Geometry: final body of the model. Coordinates: model frame, mm. Face numbers are marked on the shaded views. A direction names the side the tool comes from. Coordinates: 2 decimals unless noted, no trailing zeros. Write each loop counter-clockwise with the first axis right and the second up, starting at its lowest first coordinate (ties: lowest second). Pieces come first, ordered by that corner, then holes.
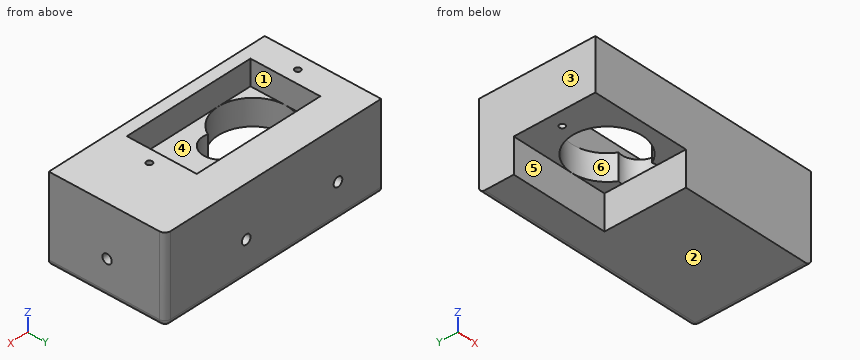
Autodesk Inventor part; units mm, degrees
ref_plane "YZ Plane" through (0, 0, 0) normal (1, 0, 0) x (0, 1, 0)
ref_plane "XZ Plane" through (0, 0, 0) normal (0, 1, 0) x (-1, 0, 0)
ref_plane "XY Plane" through (0, 0, 0) normal (0, 0, 1) x (1, 0, 0)
sketch "Sketch1" plane through (0, 0, 0) normal (0, 0, 1) x (1, 0, 0)
  line L0 (0, 0) -> (-40, 0)
  line L1 (-40, 0) -> (-40, -18)
  line L2 (-40, -18) -> (0, -18)
  line L3 (0, -18) -> (0, 0)
  dimension "d0" = 40
  dimension "d1" = 18
extrude "Extrusion1" add sketch "Sketch1" along normal blind 14.66
sketch "Sketch2" plane through (0, 0, 14.66) normal (0, 0, 1) x (1, 0, 0)
  circle A0 centre (-37.5, -12) radius 0.5
  circle A1 centre (-10, -12) radius 0.5
  line L0 (-40, -18) -> (0, -18)
  line L1 (-40, 0) -> (-40, -18)
  line L2 (-35.2, -6) -> (-12.3, -6)
  line L3 (-12.3, -6) -> (-12.3, -18)
  line L4 (-12.3, -18) -> (-35.2, -18)
  line L5 (-35.2, -18) -> (-35.2, -6)
  circle A2 centre (-29.2, -12) radius 6
  circle A3 centre (-23.2, -12) radius 3
  point P0 (0, 0)
  point P1 (-23.95, -9.0953)
  point P2 (-23.95, -14.9047)
  dimension "d4" = 1
  dimension "d5" = 1
  dimension "d6" = 6
  dimension "d7" = 6
  dimension "d8" = 27.5
  dimension "d9" = 2.5
  dimension "d10" = 12
  dimension "d11" = 4.8
  dimension "d12" = 2.3
  dimension "d17" = 6
  dimension "d18" = 6
extrude "Extrusion2" cut sketch "Sketch2" against normal blind 4.3 contours L5 A2 L0 | A2 A3 L2 L3 L0 | A2 A3 | L5 L2 A2 | A3 A2 | A2 A3
extrude "Extrusion3" cut sketch "Sketch2" against normal blind 9 contours A0 | A1
extrude "Extrusion4" cut sketch "Sketch2" against normal blind 8.75 contours A2 A3 | A3 A2 | A2 A3
sketch "Sketch3" plane through (0, 0, 5.91) normal (0, 0, 1) x (1, 0, 0)
  line L0 (-29.2, -6) -> (-12.3, -6)
  line L1 (-23.2, -6) -> (-41.4611, -6)
  line L2 (-41.4611, -6) -> (-41.4611, -19.254)
  line L3 (-41.4611, -19.254) -> (-23.2, -19.254)
  line L4 (-23.2, -19.254) -> (-23.2, -6)
  point P0 (0, 0)
  dimension "d21" = 23.2
extrude "Extrusion5" cut sketch "Sketch3" against normal blind 8.75
sketch "Sketch4" plane through (0, -18, 0) normal (0, -1, 0) x (1, 0, 0)
  line L0 (0, 0) -> (0, 14.66)
  line L1 (-23.95, 5.91) -> (-23.2, 5.91)
  line L2 (0, 0) -> (-23.2, 0)
  line L3 (-23.2, 0) -> (-23.2, 5.91)
  line L4 (-23.2, 5.91) -> (0, 5.91)
  line L5 (0, 5.91) -> (0, 0)
  line L6 (0, 14.66) -> (-40, 14.66)
  line L7 (0, 5.91) -> (-40, 5.91)
  line L8 (-40, 5.91) -> (-40, 14.66)
  line L9 (-40, 14.66) -> (0, 14.66)
  line L10 (0, 14.66) -> (0, 5.91)
extrude "Extrusion6" add sketch "Sketch4" along normal blind 2
fillet "Fillet1" radius 1 3 edges at (0, -10, 0) (-20, 0, 0) (0, 0, 7.33)
sketch "Sketch5" plane through (0, -20, 1) normal (1, 0, 0) x (0, 0, -1)
  circle A0 centre (-5, 10) radius 0.8
  line L0 (1, 0) -> (1, 19)
  line L1 (0, 0) -> (-13.66, 0)
  point P0 (1, 20)
  dimension "d27" = 1.6
  dimension "d28" = 6
  dimension "d29" = 10
extrude "Extrusion7" cut sketch "Sketch5" against normal blind 8
sketch "Sketch6" plane through (-40, 0, 1) normal (0, 1, 0) x (1, 0, 0)
  circle A0 centre (25, -5) radius 0.8
  circle A1 centre (8, -5) radius 0.8
  line L0 (39, 1) -> (0, 1)
  line L1 (40, -13.66) -> (40, 0)
  line L2 (0, 0) -> (0, -13.66)
  point P0 (40, 1)
  dimension "d32" = 1.6
  dimension "d33" = 1.6
  dimension "d34" = 6
  dimension "d35" = 6
  dimension "d36" = 15
  dimension "d37" = 8
extrude "Extrusion8" cut sketch "Sketch6" against normal blind 8 contours A0
extrude "Extrusion9" cut sketch "Sketch6" against normal blind 5.5 contours A1
equation "\"d5\" = d4"
equation "\"d6\" = 0.5 * d10"
equation "\"d7\" = d6"
equation "\"d32\" = d27"
equation "\"d33\" = d27"
properties part number "ServoMount_a"
Item 1: Set-up query: the marked faces 4, 5 and 6. Return all of +Z, -Z, +X, -X, +Y, -Y with unobstructed straight access to the full face (end or side cutting, diameter ignored); none if empty.
Derived:
face 4: +Z
face 5: -Z, -X, -Y
face 6: +Z, -Z
Item 2: Section D-D, the plane x = -10. Output: boundary loops of the cut face in (y, z).
Derived:
outline: (-20, 0) - (-1, 0) arc R1 ccw to (0, 1) - (0, 14.66) - (-11.5, 14.66) - (-11.5, 5.66) - (-12.5, 5.66) - (-12.5, 14.66) - (-20, 14.66) - close
Item 3: Section B-B, the plane x = -28. Output: boundary loops of the cut face in (y, z).
Derived:
outline: (-20, 5.91) - (-17.88, 5.91) - (-17.88, 10.36) - (-18, 10.36) - (-18, 14.66) - (-20, 14.66) - close; (-6.12, 5.91) - (-6, 5.91) - (-6, 0) - (-1, 0) arc R1 ccw to (0, 1) - (0, 14.66) - (-6, 14.66) - (-6, 10.36) - (-6.12, 10.36) - close
Item 4: Pin query (flat end, axial travel): pin 1 (0.5 mm diameter, centred on x = -10, y = -12, fed in from +Z); pin 2 (0.5 mm diameter, centred on x = -15, z = 6, fed in from +Y); pin 3 (0.9 mm diameter, centred on x = -21, y = -12.5, fed in from +Z); pin 4 (5 mm diameter, centred on x = -31.5, y = -10.5, fed in from +Z). Return the tip coordinate at first contact, or that it passes through.
Derived:
pin 1: stops at z = 5.66
pin 2: stops at y = -8
pin 3: stops at z = 5.91
pin 4: passes through
Item 5: Material intervals for probe 1 along X at (y, z) = (-8, 11.25); probe 2 along Z at (x, y) = (-32, -2.85); probe 3 along Y at (x, z) = (-19, 11.75), sorted ascending.
Derived:
probe 1: x = -40 to -35.2, -12.3 to 0
probe 2: z = 0 to 5.2, 6.8 to 14.66
probe 3: y = -20 to -18, -6 to 0
Item 6: Pull-direction query (X, two-part tool) for the marked faces 1, 2 and 3; classes: released by +X, released by -X, zero draft, split by the parting line, or undercut.
Derived:
face 1: undercut
face 2: zero draft
face 3: released by -X
Item 7: Section C-C, the plane y = -16.5. Output: boundary loops of the cut face in (x, z).
Derived:
outline: (-40, 5.91) - (-33.17, 5.91) - (-33.17, 10.36) - (-35.2, 10.36) - (-35.2, 14.66) - (-40, 14.66) - close; (-25.23, 5.91) - (-23.2, 5.91) - (-23.2, 0) - (-1, 0) arc R1 ccw to (0, 1) - (0, 14.66) - (-12.3, 14.66) - (-12.3, 10.36) - (-25.23, 10.36) - close
Item 8: Section A-A, the plane z = 10.75. Output: boundary loops of the cut face in (x, y), plus the area to 3 significant figures.
Derived:
outline: (-40, -20) - (0, -20) - (0, -1) arc R1 ccw to (-1, 0) - (-40, 0) - close; hole circle Ø1 at (-37.5, -12); hole (-35.2, -18) - (-12.3, -18) - (-12.3, -6) - (-35.2, -6) - close; hole circle Ø1 at (-10, -12)
area: 523 mm2
